from build123d import *

# Parameters (mm, degrees)
F0_W           = 107.3
F0_H           = 6.35
F1_DEPTH       = 6.35
F2_R           = 3
F4_D           = 2.0574
F4_CSINK_D     = 4.2672
F4_CSINK_ANGLE = 82


with BuildPart() as f1:
    # F0 (on Top) → F1 (new body)
    with BuildSketch(Plane.XY):
        Rectangle(F0_W, F0_H)
    extrude(amount=F1_DEPTH)

    # F2
    f2_edges = [f1.edges().sort_by_distance(p)[0] for p in [
        (0, 3.175, 6.35),
        (0, -3.175, 6.35),
    ]]
    fillet(f2_edges, radius=F2_R)

    # F4 (through all)
    with Locations(Plane.XY.offset(6.35)):
        with Locations((-14.9764604867, 0), (15.0013882667, 0), (44.9633300304, 0), (-45.0155586004, 0)):
            CounterSinkHole(F4_D / 2, F4_CSINK_D / 2, counter_sink_angle=F4_CSINK_ANGLE)


solid = f1.part
Input: part model. Units: mm. Frame: model coordinates. Coordinates: 2 decimals unless noted, no trailing zeros. Loops run counter-clockwise (first coordinate to the right, second up) from the corner with the lowest first, then second, coordinate; pieces in that order, holes last.
(1) Section A-A on x = 20.5. Return the cut outline in (y, z) (3 decimals).
(2) Pull-direction query (X, two-part tool) for faces 1 (the face through (0.75, 2.32, 5.45)), 2 (the face through (53.65, 0, 3)), 3 (the face through (44.01, -0.39, 2.5)); classes: released by +X, released by -X, zero draft, split by the parting line, or undercut.
(3) Material intervals for probe 1 along X at (y, z) = (0, 2.9); probe 2 along X at (y, z) = (0.5, 2); probe 3 along Y at (x, z) = (-23, 3.5), sorted ascending.
(4) First-contact query: pin 1 Ø3.5 at (x, y) = (44.96, 0) entering from +Z; pin 2 Ø1.5 at (x, y) = (-32, -1.5) entering from +Z. Flat tips, straight axial feed; report the tip coordinate or a pass-through.
Data:
1. outline: (-3.175, 0) - (3.175, 0) - (3.175, 3.35) arc R3 ccw to (0.175, 6.35) - (-0.175, 6.35) arc R3 ccw to (-3.175, 3.35) - close
2. face 1: zero draft
2. face 2: released by +X
2. face 3: undercut
3. probe 1: x = -53.65 to -46.04, -43.99 to -16.01, -13.95 to 13.97, 16.03 to 43.93, 45.99 to 53.65
3. probe 2: x = -53.65 to -45.91, -44.12 to -15.88, -14.08 to 14.1, 15.9 to 44.06, 45.86 to 53.65
3. probe 3: y = -3.17 to 3.17
4. pin 1: stops at z = 5.91
4. pin 2: stops at z = 6.29
